from build123d import *

# Parameters (mm, degrees)
SKETCH4_R                = 2.75
CUT_EXTRUDE4_DEPTH       = 3
SKETCH5_OUTSIDE_W        = 33.422
SKETCH5_OUTSIDE_H        = 33.422
CUT_EXTRUDE5_DEPTH       = 20.697715604
CUT_EXTRUDE2_DEPTH       = 10
BOSS_EXTRUDE1_REACH      = 27.298
BOSS_EXTRUDE1_END_RADIUS = 5
SKETCH3_R                = 2.75
CUT_EXTRUDE6_REACH       = 27.298
SKETCH6_R                = 1.6
FILLET1_R                = 0.5
CHAMFER1_SIZE            = 0.5
FILLET2_R                = 1
SKETCH7_R                = 1.55
CUT_EXTRUDE7_DEPTH       = 20.025404425


with BuildPart() as part:
    # Sketch1 → Revolve1 (revolve)
    with BuildSketch(Plane(origin=(0, 0, 0), x_dir=(0, 0, -1), z_dir=(1, 0, 0))):
        Polygon((0, 0), (12, 0), (12, 5), (5, 5), (5, 15), (0, 15), (0, 5.353547723), align=None)
    revolve(axis=Axis((0, 5.353547723, 0), (0, 1, 0)))

    # Sketch4 → Cut-Extrude4 (cut)
    with BuildSketch(Plane(origin=(0, 5, 0), x_dir=(1, 0, 0), z_dir=(0, 1, 0))):
        with Locations(Location((0, 8.5, 0), (0, 0, 270))):
            Circle(SKETCH4_R)
        with Locations(Location((7.361215932, -4.25, 0), (0, 0, 270))):
            Circle(SKETCH4_R)
        with Locations(Location((-7.361215932, -4.25, 0), (0, 0, 270))):
            Circle(SKETCH4_R)
    extrude(amount=-CUT_EXTRUDE4_DEPTH, mode=Mode.SUBTRACT)

    # Sketch5 outside → Cut-Extrude5 (cut, through all)
    with BuildSketch(Plane(origin=(0, 5, 0), x_dir=(1, 0, 0), z_dir=(0, 1, 0))):
        Rectangle(SKETCH5_OUTSIDE_W, SKETCH5_OUTSIDE_H)
        with BuildLine():
            Line((-3.031088913, 10.25), (-10.392304845, -2.5))
            ThreePointArc((-10.392304845, -2.5), (-10.392304845, -6), (-7.361215932, -7.75))
            Line((-7.361215932, -7.75), (7.361215932, -7.75))
            ThreePointArc((7.361215932, -7.75), (10.392304845, -6), (10.392304845, -2.5))
            Line((10.392304845, -2.5), (3.031088913, 10.25))
            ThreePointArc((3.031088913, 10.25), (0, 12), (-3.031088913, 10.25))
        make_face(mode=Mode.SUBTRACT)
    extrude(amount=-CUT_EXTRUDE5_DEPTH, mode=Mode.SUBTRACT)

    # Sketch2 → Cut-Extrude2 (cut)
    with BuildSketch(Plane(origin=(0, 15, 0), x_dir=(1, 0, 0), z_dir=(0, 1, 0))):
        Polygon((2.944486373, 0), (1.472243186, 2.55), (-1.472243186, 2.55), (-2.944486373, 0), (-1.472243186, -2.55), (1.472243186, -2.55), align=None)
    extrude(amount=-CUT_EXTRUDE2_DEPTH, mode=Mode.SUBTRACT)

    # Boss-Extrude1: up to this cylinder (the profile starts outside it)
    boss_extrude1_end = Plane(origin=(0, 10, 0), z_dir=(0, -1, 0)) * Cylinder(BOSS_EXTRUDE1_END_RADIUS, 65.596, mode=Mode.PRIVATE)
    # Sketch3 → Boss-Extrude1 (add, up to the surface)
    with BuildSketch(Plane(origin=(6.105479097, 0, -3.525), x_dir=(-0.5000000000000001, 0, -0.8660254037844386), z_dir=(0.8660254037844386, 0, -0.5000000000000001)), mode=Mode.PRIVATE) as boss_extrude1_sk1:
        with Locations((0, 10)):
            Circle(SKETCH3_R)
    boss_extrude1_tool1 = extrude(boss_extrude1_sk1.sketch, amount=-BOSS_EXTRUDE1_REACH, mode=Mode.PRIVATE) - boss_extrude1_end
    add(boss_extrude1_tool1.solids().sort_by_distance((6.105479, 10, -3.525))[0])

    # Sketch6 → Cut-Extrude6 (cut, up to next)
    with BuildSketch(Plane(origin=(6.105479097, 0, -3.525), x_dir=(-0.5000000000000001, 0, -0.8660254037844386), z_dir=(0.8660254037844386, 0, -0.5000000000000001)), mode=Mode.PRIVATE) as cut_extrude6_sk1:
        with Locations((0, 10)):
            Circle(SKETCH6_R)
    cut_extrude6_tool1 = extrude(cut_extrude6_sk1.sketch, amount=-CUT_EXTRUDE6_REACH, mode=Mode.PRIVATE) & part.part
    add(cut_extrude6_tool1.solids().sort_by_distance((6.105479, 10, -3.525))[0], mode=Mode.SUBTRACT)

    # Fillet1
    fillet1_edges = [part.edges().sort_by_distance(p)[0] for p in [
        (0, 5, 5),
    ]]
    fillet(fillet1_edges, radius=FILLET1_R)

    # Chamfer1
    chamfer1_edges = [part.edges().sort_by_distance(p)[0] for p in [
        (6.905479097, 10, -2.139359354),
    ]]
    chamfer(chamfer1_edges, length=CHAMFER1_SIZE)

    # Fillet2
    fillet2_edges = [part.edges().sort_by_distance(p)[0] for p in [
        (4.991369035, 9.999999998, 0.293658225),
    ]]
    fillet(fillet2_edges, radius=FILLET2_R)

    # Sketch7 → Cut-Extrude7 (cut, through all)
    with BuildSketch(Plane(origin=(0, 5, 0), x_dir=(1, 0, 0), z_dir=(0, 1, 0))):
        with Locations(Location((0, 8.5, 0), (0, 0, 270))):
            Circle(SKETCH7_R)
        with Locations(Location((7.361215932, -4.25, 0), (0, 0, 270))):
            Circle(SKETCH7_R)
        with Locations(Location((-7.361215932, -4.25, 0), (0, 0, 270))):
            Circle(SKETCH7_R)
    extrude(amount=-CUT_EXTRUDE7_DEPTH, mode=Mode.SUBTRACT)


solid = part.part
Can you work these out from the model? Positions are in its coordinate system, mm. A direction names the side the tool comes from. Coordinates: 2 decimals unless noted, no trailing zeros. Write each loop counter-clockwise with the first axis right and the second up, starting at its lowest first coordinate (ties: lowest second). Pieces come first, ordered by that corner, then holes. Notation, with made-up numbers: M -32,-39.75 L 1,-39.75 A25 ccw 1,-9.75 Z; hole C -9.75,7 d5. An arc over 180 degrees is marked long. Use one line per item in the form item = value.
Q1. If we section it at A-A (x = 0): Write out the boundary of the cut face in (y, z).
Model answer:
outline = M 0,-12 L 5,-12 L 5,-11.25 L 2,-11.25 L 2,-10.05 L 0,-10.05 Z; M 0,-6.95 L 2,-6.95 L 2,-5.75 L 5,-5.75 L 5,-5.5 A0.5 cw 5.5,-5 L 15,-5 L 15,-2.55 L 5,-2.55 L 5,2.55 L 15,2.55 L 15,5 L 5.5,5 A0.5 cw 5,5.5 L 5,7.75 L 0,7.75 Z
Q2. For faces 1 (the flat face through (-2.219, 10.07, 1.257)), 2 (the cylindrical face through (6.42, 1.01, 3.02)), which set-ups out of +Z, -Z, +X, -X, +Y, -Y let a thin tool reach every point of the face, with its end or its side?
Model answer:
face_1 = +Y
face_2 = +Y, -Y
Q3. For P1, Ø1.5, axis at x = 0, y = 10, coming from the -Z side; P2, Ø6, axis at x = 8.5, y = 10.5, coming from the +Z side; P3, Ø4, axis at x = 4, y = 11.5, coming from the -Z side, each with a flat end and sliding along its axis, tell me the tip position at first contact or that it passes through.
Model answer:
P1 = -5
P2 = -0.02
P3 = -5.91
Q4. If we section it at B-B (y = 4): Write out the boundary of the cut face in (x, z), then the cut area to 3 significant figures.
Model answer:
outline = M -10.39,2.5 L -3.03,-10.25 A3.5 ccw 3.03,-10.25 L 10.39,2.5 A3.5 ccw 7.36,7.75 L -7.36,7.75 A3.5 ccw Z; hole C -7.36,4.25 d5.5; hole C 0,-8.5 d5.5; hole C 7.36,4.25 d5.5
area = 216 mm^2
Q5. If we section it at D-D (x = 9.5): Write out the boundary of the cut face in (y, z), then the cut area to 3 significant figures.
Model answer:
outline = M 0,0.95 L 5,0.95 L 5,2.52 L 2,2.52 L 2,5.98 L 5,5.98 L 5,7.02 L 0,7.02 Z
area = 20.0 mm^2
Q6. I need wall thicknesses on line 1 along Y through (x, z) = (5.5, -3.5); line 2 along Y through (x, z) = (-1.5, -6.25); line 3 along X through (y, z) = (2.9, -8.5). Which ranges of each line are inside material? Lowest first, please. Write a range as from..to.
Model answer:
line_1 = 0..5, 7.26..8.42, 11.58..12.74
line_2 = 0..2
line_3 = -4.04..-2.75, 2.75..4.04
Q7. If we section it at C-C (z = -7.75): Write out the boundary of the cut face in (x, y).
Model answer:
outline = M -4.47,0 L -1.36,0 L -1.36,2 L -2.65,2 L -2.65,5 L -4.47,5 Z; M 1.36,0 L 4.47,0 L 4.47,5 L 2.65,5 L 2.65,2 L 1.36,2 Z
Q8. We'd pull the mould along X, two halves only. Please class faces 3 (the flat face through (-6.66, 2.535, -3.964)), 4 (the flat face through (0, 0, 0)), 5 (the flat face through (-9, 2, 5)): +X half, -X half, draft (parallel to the pull), parting line (faces both ways), or undercut.
Model answer:
face_3 = -X half
face_4 = draft
face_5 = undercut
